Can you work these out from the model? Positions are in its coordinate system, mm. A direction names the side the tool comes from. Round coordinates to 2 decimals unless told otherwise and drop trailing zeros. Order: outer loops, then holes, each group sorted by start corner. A loop starts at its lowest first (then second) coordinate and runs counter-clockwise, first axis right, second up. Notation, with made-up numbers: M 38.25,18.25 L 48.25,18.25 A7 cw 48.25,24.25 Z; hole C -31,74.25 d6. An arc over 180 degrees is marked long. One line per question, with ' | ' between items.
```python
from build123d import *

# Parameters (mm, degrees)
F2_DEPTH = 750


with BuildPart() as f2:
    # F1 (on face) → F2 (new body)
    with BuildSketch(Plane.XY):
        with BuildLine():
            ThreePointArc((19.8, -30.3), (20.153553, -30.153553), (20.3, -29.8))
            Line((20.3, -29.8), (20.3, 29.8))
            ThreePointArc((20.3, 29.8), (20.153553, 30.153553), (19.8, 30.3))
            Line((19.8, 30.3), (6, 30.3))
            ThreePointArc((6, 30.3), (5.646447, 30.153553), (5.5, 29.8))
            Line((5.5, 29.8), (5.5, 22.8))
            ThreePointArc((5.5, 22.8), (5.353553, 22.446447), (5, 22.3))
            Line((5, 22.3), (-5, 22.3))
            ThreePointArc((-5, 22.3), (-5.353553, 22.446447), (-5.5, 22.8))
            Line((-5.5, 22.8), (-5.5, 29.8))
            ThreePointArc((-5.5, 29.8), (-5.646447, 30.153553), (-6, 30.3))
            Line((-6, 30.3), (-19.8, 30.3))
            ThreePointArc((-19.8, 30.3), (-20.153553, 30.153553), (-20.3, 29.8))
            Line((-20.3, 29.8), (-20.3, -29.8))
            ThreePointArc((-20.3, -29.8), (-20.153553, -30.153553), (-19.8, -30.3))
            Line((-19.8, -30.3), (-6, -30.3))
            ThreePointArc((-6, -30.3), (-5.646447, -30.153553), (-5.5, -29.8))
            Line((-5.5, -29.8), (-5.5, -22.8))
            ThreePointArc((-5.5, -22.8), (-5.353553, -22.446447), (-5, -22.3))
            Line((-5, -22.3), (5, -22.3))
            ThreePointArc((5, -22.3), (5.353553, -22.446447), (5.5, -22.8))
            Line((5.5, -22.8), (5.5, -29.8))
            ThreePointArc((5.5, -29.8), (5.646447, -30.153553), (6, -30.3))
            Line((6, -30.3), (19.8, -30.3))
        make_face()
        with BuildLine():
            Line((5, -19.8), (-5, -19.8))
            ThreePointArc((-5, -19.8), (-7.12132, -20.67868), (-8, -22.8))
            Line((-8, -22.8), (-8, -27.8))
            Line((-8, -27.8), (-17.8, -27.8))
            Line((-17.8, -27.8), (-17.8, 27.8))
            Line((-17.8, 27.8), (-8, 27.8))
            Line((-8, 27.8), (-8, 22.8))
            ThreePointArc((-8, 22.8), (-7.12132, 20.67868), (-5, 19.8))
            Line((-5, 19.8), (5, 19.8))
            ThreePointArc((5, 19.8), (7.12132, 20.67868), (8, 22.8))
            Line((8, 22.8), (8, 27.8))
            Line((8, 27.8), (17.8, 27.8))
            Line((17.8, 27.8), (17.8, -27.8))
            Line((17.8, -27.8), (8, -27.8))
            Line((8, -27.8), (8, -22.8))
            ThreePointArc((8, -22.8), (7.12132, -20.67868), (5, -19.8))
        make_face(mode=Mode.SUBTRACT)
    extrude(amount=F2_DEPTH)


solid = f2.part
```
(1) Will these pins go through, and if not, where does the flat tip stop? pin 1 Ø5 at (x, z) = (-1, 375.5) entering from +Y; pin 2 Ø3 at (x, z) = (-2.5, 392) entering from -Y; pin 3 Ø8 at (x, z) = (2, 425.5) entering from +Y; pin 4 Ø10 at (x, y) = (3, 14) entering from -Z.
Final values:
pin 1: y = 22.3 | pin 2: y = -22.3 | pin 3: y = 30.3 | pin 4: through
(2) If we section it at A-A on y = -1: Please give me the cut outline in (x, z).
Final values:
outline: M -20.3,0 L -17.8,0 L -17.8,750 L -20.3,750 Z; M 17.8,0 L 20.3,0 L 20.3,750 L 17.8,750 Z
(3) On a 3-axis mill with a long thin cutter (end or side, diameter ignored), from which of +Z, -Z, +X, -X, +Y, -Y can I reach the whole of each face in a straight line? I mean faces 5 (the flat face through (17.8, 0, 370)), 6 (the flat face through (-18, 0, 750)). Say none if no direction works.
Final values:
face 5: +Z, -Z | face 6: +Z, +X, -X, +Y, -Y
(4) Please list where these lines run through material, in increasing order: probe 1 along X at (y, z) = (25.5, 138); probe 2 along Y at (x, z) = (0, 605); probe 3 along Y at (x, z) = (15.5, 69). Write a range as [from, to].
Final values:
probe 1: [-20.3, -17.8], [-8, -5.5], [5.5, 8], [17.8, 20.3] | probe 2: [-22.3, -19.8], [19.8, 22.3] | probe 3: [-30.3, -27.8], [27.8, 30.3]
(5) Thinking about a two-plate mould opening in X: for faces 1 (the flat face through (-17.8, 0, 370)), 2 (the flat face through (20.3, 0, 370)), 3 (the flat face through (-20.3, 0, 370)), 4 (the flat face through (-13, -30.3, 370)), which applies, released by +X, released by -X, zero draft, split by the parting line, or undercut?
Final values:
face 1: undercut | face 2: released by +X | face 3: released by -X | face 4: zero draft
